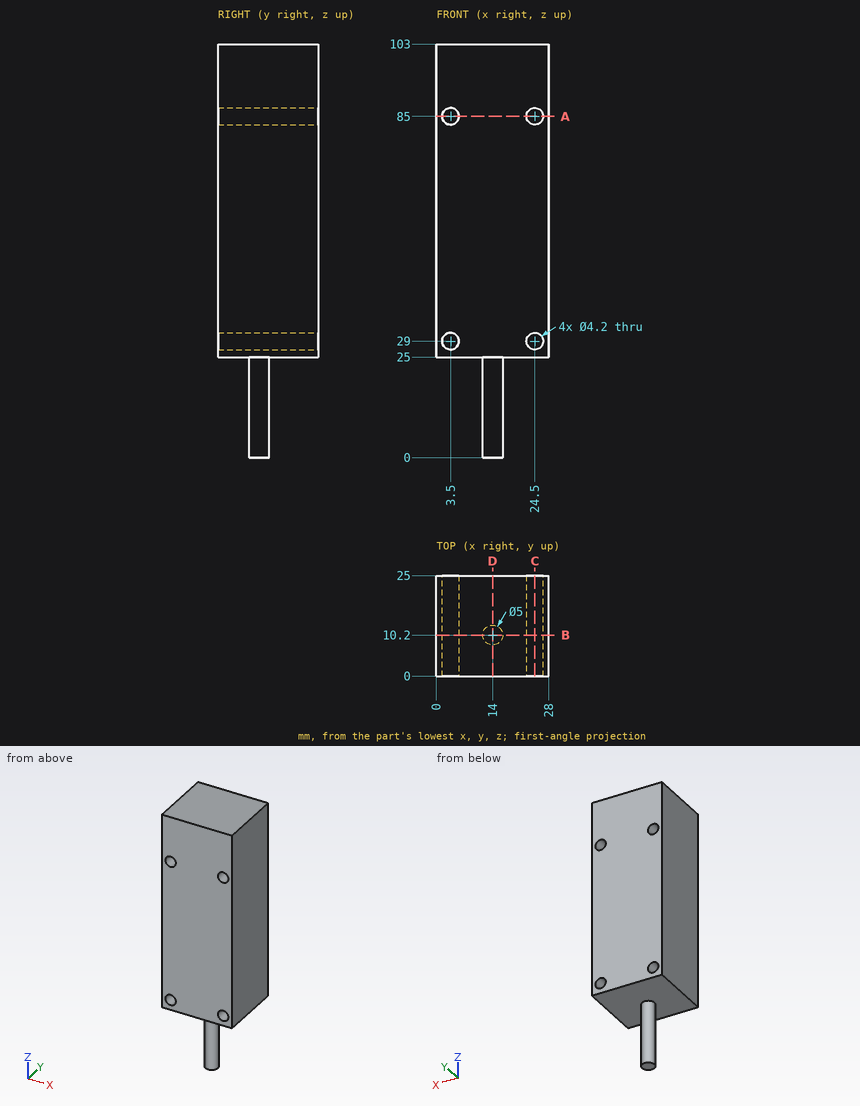
Study the drawing (mm; zero at the part's minimum x, y, z) and answer. Coordinates: 2 decimals unless noted, no trailing zeros. Write each loop counter-clockwise with the first axis right and the second up, starting at its lowest first coordinate (ties: lowest second). Pieces come first, ordered by that corner, then holes. Notation, with made-up numbers: M 39,-16 L 94,-16 A30 cw 94,15 Z; hole C 13,26.5 d6. An arc over 180 degrees is marked long. Use a Markdown table: item, result. Add a question column.
1. Section A-A (z = 85) is taken. Give the vertices of the cut face in (x, y), plus the area to 3 significant figures.
2. Section C-C (x = 24.5) is taken. Give the vertices of the cut face in (y, z).
3. Straight lines are drawn through the part: line 1 along Z through (x, y) = (3.5, 8.25); line 2 along Z through (x, y) = (24, 22.5); line 3 along Z through (x, y) = (14, 13.75). For each, find the intervals that lie inside material, in ascending order. Write a range as [from, to].
4. Section D-D (x = 14) is taken. Give the vertices of the cut face in (y, z), plus the area to 4 significant figures.
5. Given P1, Ø8, axis at x = 18.5, y = 21, coming from the -Z side, flat-ended and moving along its own axis, determine where the tip first touches the part or whether it passes through.
6. Section B-B (y = 10.2) is taken. Give the vertices of the cut face in (x, z), plus the area to 3 significant figures.
Data:
| question | item | result |
|---|---|---|
| 1 | outline | M 0,0 L 1.4,0 L 1.4,25 L 0,25 Z; M 5.6,0 L 22.4,0 L 22.4,25 L 5.6,25 Z; M 26.6,0 L 28,0 L 28,25 L 26.6,25 Z |
| 1 | area | 490 mm2 |
| 2 | outline | M 0,25 L 25,25 L 25,26.9 L 0,26.9 Z; M 0,31.1 L 25,31.1 L 25,82.9 L 0,82.9 Z; M 0,87.1 L 25,87.1 L 25,103 L 0,103 Z |
| 3 | line 1 | z = [25, 26.9], [31.1, 82.9], [87.1, 103] |
| 3 | line 2 | z = [25, 26.96], [31.04, 82.96], [87.04, 103] |
| 3 | line 3 | z = [25, 103] |
| 4 | outline | M 0,25 L 7.7,25 L 7.7,0 L 12.7,0 L 12.7,25 L 25,25 L 25,103 L 0,103 Z |
| 4 | area | 2,075 mm2 |
| 5 | P1 | stops at z = 25 |
| 6 | outline | M 0,25 L 11.5,25 L 11.5,0 L 16.5,0 L 16.5,25 L 28,25 L 28,103 L 0,103 Z; hole C 3.5,29 d4.2; hole C 3.5,85 d4.2; hole C 24.5,29 d4.2; hole C 24.5,85 d4.2 |
| 6 | area | 2,250 mm2 |
